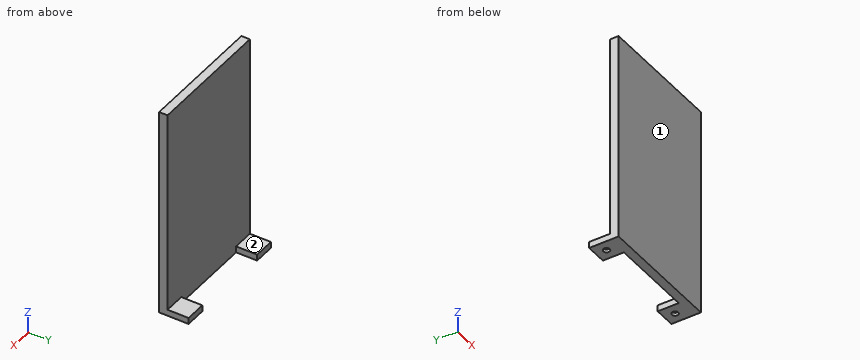
Autodesk Inventor part; units mm, degrees
ref_plane "YZ Plane" through (0, 0, 0) normal (1, 0, 0) x (0, 1, 0)
ref_plane "XZ Plane" through (0, 0, 0) normal (0, 1, 0) x (-1, 0, 0)
ref_plane "XY Plane" through (0, 0, 0) normal (0, 0, 1) x (1, 0, 0)
sketch "草圖1" plane through (0, 0, 0) normal (0, 0, 1) x (1, 0, 0)
  line L0 (0, 0) -> (10, 0)
  line L1 (10, 0) -> (10, 10)
  line L2 (10, 10) -> (0, 10)
  line L3 (0, 10) -> (0, 0)
  circle A0 centre (5, 5) radius 1.5
  point P0 (5, 10)
  point P1 (10, 5)
  dimension "d0" = 10
  dimension "d1" = 10
  dimension "d2" = 3
extrude "擠出1" add sketch "草圖1" along normal blind 3 contours L3 L2 L1 L0 | A0
extrude "擠出2" cut sketch "草圖1" along normal blind 1.5 contours A0
sketch "草圖2" plane through (0, 0, 0) normal (0, 1, 0) x (-1, 0, 0)
  line L0 (0, 0) -> (-60, 0)
  line L1 (-60, 0) -> (-60, 100)
  line L2 (-60, 100) -> (0, 100)
  line L3 (0, 100) -> (0, 0)
  dimension "d7" = 60
  dimension "d8" = 100
pattern_linear "矩形陣列1" count 2 spacing 50 along (1, 0, 0) of "擠出2", "擠出1"
extrude "擠出3" add sketch "草圖2" against normal blind 4
properties part number "110033226_ipt_42_城堡門口橋"
Source: CAD feature listing. Evaluate the final solid. Frame: model axes, mm. Face numbers are marked on the shaded views. A direction names the side the tool comes from. Coordinates: 2 decimals unless noted, no trailing zeros. Loops run counter-clockwise (first coordinate to the right, second up) from the corner with the lowest first, then second, coordinate; pieces in that order, holes last. Notation, with made-up numbers: M 15.5,40.25 L 24.5,40.25 A9 cw 24.5,49.25 Z; hole C 83,-0.75 d9. An arc over 180 degrees is marked long. Use a Markdown table: item, result. Add a question column.
Q1. Access query for the marked faces 1 and 2. Directions: +Z, -Z, +X, -X, +Y, -Y. A direction counts if a zero-diameter tool reaches every point of the face in a straight line with its end or side. Return the directions, or none.
Q2. Section query A-A, the plane y = 5. Return loops of the section in (x, z).
Q3. First-contact query: pin 1 (8 mm diameter, centred on x = 23.5, z = 67.5, fed in from +Y); pin 2 (1.5 mm diameter, centred on y = 1.5, z = 40.5, fed in from +X); pin 3 (2.5 mm diameter, centred on x = 55, y = 5, fed in from -Z). Flat tips, straight axial feed; report the tip coordinate or a pass-through.
Q4. Material intervals for L1, parallel to Y at x = 55, z = 0.95; L2, parallel to Y at x = 51.5, z = 29; L3, parallel to Z at x = 55.5, y = 7.75, sorted ascending.
Q5. Section query B-B, the plane x = 55. Return loops of the section in (y, z), and give its area (4 significant figures).
Q6. Section query C-C, the plane z = 44. Return loops of the section in (x, y), and give its area (3 significant figures).
Q7. Section query D-D, the plane x = 20.5. Return loops of the section in (y, z), and give its area (3 significant figures).
Result:
| question | item | result |
|---|---|---|
| 1 | face 1 | +Z, -Z, +X, -X, -Y |
| 1 | face 2 | +Z, +X, -X, +Y |
| 2 | outline | M 0,0 L 3.5,0 L 3.5,1.5 L 6.5,1.5 L 6.5,0 L 10,0 L 10,3 L 0,3 Z; M 50,0 L 53.5,0 L 53.5,1.5 L 56.5,1.5 L 56.5,0 L 60,0 L 60,3 L 50,3 Z |
| 3 | pin 1 | stops at y = 0 |
| 3 | pin 2 | passes through |
| 3 | pin 3 | stops at z = 1.5 |
| 4 | L1 | y = -4 to 3.5, 6.5 to 10 |
| 4 | L2 | y = -4 to 0 |
| 4 | L3 | z = 0 to 3 |
| 5 | outline | M -4,0 L 3.5,0 L 3.5,1.5 L 6.5,1.5 L 6.5,0 L 10,0 L 10,3 L 0,3 L 0,100 L -4,100 Z |
| 5 | area | 425.5 mm2 |
| 6 | outline | M 0,-4 L 60,-4 L 60,0 L 0,0 Z |
| 6 | area | 240 mm2 |
| 7 | outline | M -4,0 L 0,0 L 0,100 L -4,100 Z |
| 7 | area | 400 mm2 |
